Read the model definition and answer for the solid it produces. Units are mm, in the model's axes. A direction names the side the tool comes from. Round coordinates to 2 decimals unless told otherwise and drop trailing zeros. Order: outer loops, then holes, each group sorted by start corner. A loop starts at its lowest first (then second) coordinate and runs counter-clockwise, first axis right, second up. Notation, with made-up numbers: M 78,85.5 L 130,85.5 A18 ccw 130,114.5 Z; hole C 44.25,4 d4. An arc over 180 degrees is marked long. Use one line per item in the form item = value. Start each with the question number.
from build123d import *

# Parameters (mm, degrees)
BOSS_EXTRUDE1_DEPTH     = 5
CUT_EXTRUDE2_DEPTH      = 1
CUT_EXTRUDE2_DEPTH_BACK = 1
FILLET1_R               = 1
BOSS_EXTRUDE3_DEPTH     = 10
FILLET2_R               = 0.8


with BuildPart() as part:
    # Sketch1 → Boss-Extrude1 (new body)
    with BuildSketch(Plane(origin=(0, 0, 0), x_dir=(1, 0, 0), z_dir=(0, 1, 0))):
        with BuildLine():
            Line((-3.9, 3.9), (0, 3.9))
            ThreePointArc((0, 3.9), (2.757716447, 2.757716447), (3.9, 0))
            Line((3.9, 0), (3.9, -3.9))
            Line((3.9, -3.9), (0, -3.9))
            ThreePointArc((0, -3.9), (-2.757716447, -2.757716447), (-3.9, 0))
            Line((-3.9, 0), (-3.9, 3.9))
        make_face()
    extrude(amount=BOSS_EXTRUDE1_DEPTH)

    # Sketch3 → Cut-Extrude2 (cut, two sides: drawn at the far end of the back side and taken through both)
    with BuildSketch(Plane(origin=(0, 2.5, 0), x_dir=(1, 0, 0), z_dir=(0, 1, 0)).offset(-CUT_EXTRUDE2_DEPTH_BACK)):
        with BuildLine():
            Line((-3.9, 0), (-3.9, 3.9))
            Line((-3.9, 3.9), (0, 3.9))
            ThreePointArc((0, 3.9), (2.757716447, 2.757716447), (3.9, 0))
            Line((3.9, 0), (3.9, -3.9))
            Line((3.9, -3.9), (0, -3.9))
            ThreePointArc((0, -3.9), (-2.757716447, -2.757716447), (-3.9, 0))
        make_face()
        with BuildLine():
            Line((-2.9, 0), (-2.9, 2.9))
            Line((-2.9, 2.9), (0, 2.9))
            ThreePointArc((0, 2.9), (2.050609665, 2.050609665), (2.9, 0))
            Line((2.9, 0), (2.9, -2.9))
            Line((2.9, -2.9), (0, -2.9))
            ThreePointArc((0, -2.9), (-2.050609665, -2.050609665), (-2.9, 0))
        make_face(mode=Mode.SUBTRACT)
    extrude(amount=CUT_EXTRUDE2_DEPTH + CUT_EXTRUDE2_DEPTH_BACK, mode=Mode.SUBTRACT)

    # Fillet1
    fillet1_edges = [part.edges().sort_by_distance(p)[0] for p in [
        (2.9, 3.5, 1.45),
        (2.050609665, 3.5, -2.050609665),
        (1.45, 3.5, 2.9),
        (-2.050609665, 3.5, 2.050609665),
        (2.9, 1.5, 1.45),
        (2.050609665, 1.5, -2.050609665),
        (-2.9, 1.5, -1.45),
        (1.45, 1.5, 2.9),
        (-1.45, 3.5, -2.9),
        (-2.9, 3.5, -1.45),
        (-1.45, 1.5, -2.9),
        (-2.050609665, 1.5, 2.050609665),
    ]]
    fillet(fillet1_edges, radius=FILLET1_R - 0.0001)  # a hair under: the kernel refuses the full size

    # Sketch4 → Boss-Extrude3 (add)
    with BuildSketch(Plane(origin=(0, 5, 0), x_dir=(1, 0, 0), z_dir=(0, 1, 0))):
        with BuildLine():
            Line((0, 3.9), (-3.9, 3.9))
            Line((-3.9, 3.9), (-3.9, 0))
            ThreePointArc((-3.9, 0), (-2.757716447, -2.757716447), (0, -3.9))
            Line((0, -3.9), (3.9, -3.9))
            Line((3.9, -3.9), (3.9, 0))
            ThreePointArc((3.9, 0), (2.757716447, 2.757716447), (0, 3.9))
        make_face()
        with BuildLine():
            Line((-2.2627417, -0.565685425), (-0.565685425, -2.2627417))
            ThreePointArc((-0.565685425, -2.2627417), (0, -2.497056275), (0.565685425, -2.2627417))
            Line((0.565685425, -2.2627417), (2.2627417, -0.565685425))
            ThreePointArc((2.2627417, -0.565685425), (2.497056275, 0), (2.2627417, 0.565685425))
            Line((2.2627417, 0.565685425), (0.565685425, 2.2627417))
            ThreePointArc((0.565685425, 2.2627417), (0, 2.497056275), (-0.565685425, 2.2627417))
            Line((-0.565685425, 2.2627417), (-2.2627417, 0.565685425))
            ThreePointArc((-2.2627417, 0.565685425), (-2.497056275, 0), (-2.2627417, -0.565685425))
        make_face(mode=Mode.SUBTRACT)
    extrude(amount=BOSS_EXTRUDE3_DEPTH)

    # Fillet2
    fillet2_edges = [part.edges().sort_by_distance(p)[0] for p in [
        (0, 15, 2.497056275),
        (1.414213562, 15, 1.414213562),
        (2.497056275, 15, 0),
        (1.414213562, 15, -1.414213562),
        (0, 15, -2.497056275),
        (-1.414213562, 15, -1.414213562),
        (-2.497056275, 15, 0),
        (-1.414213562, 15, 1.414213562),
    ]]
    fillet(fillet2_edges, radius=FILLET2_R)


solid = part.part
Item 1: A tool of negligible diameter and unlimited length cuts with its end or side. For faces 4 (the cylindrical face through (3.201, 1.785, 1.544)), 5 (the cylindrical face through (-3.185, 3.199, -1.544)), 6 (the cylindrical face through (1.596, 14.772, 1.572)), from which of +Z, -Z, +X, -X, +Y, -Y can it reach the whole face along a straight path? Write none if from no direction.
Item 2: Find the intervals of material crossed by L1, parallel to Y at x = -3.5, z = -1.5; L2, parallel to X at y = 8.5, z = -0.25; L3, parallel to Y at x = -1.5, z = 2.75, in increasing order. Write a range as [from, to].
Item 3: Given P1, Ø2.5, axis at x = 0, z = -1, coming from the +Y side; P2, Ø1.5, axis at x = 1.5, z = -0.5, coming from the +Y side, each flat-ended and moving along its own axis, determine where each tip first touches the part or whether it passes through.
Item 4: Section A-A (y = 7.75) is taken. Write down the section's boundary in (x, z).
Item 5: Section B-B (y = 3) is taken. Write down the section's boundary in (x, z).
Item 6: For a pull along Z with two mould halves and no side action, classify faces 1 (the flat face through (-2, 9, -3.9)), 2 (the flat face through (-1.43, 9.54, 1.4)), 3 (the flat face through (-3.9, 1, -2)) as pulls with the +Z half, pulls with the -Z half, needs draft (parallel to the pull), parting line crosses it, or undercut.
The answers:
q1.face_4 = +Z, -Z, +X
q1.face_5 = +Z, -Z, -X
q1.face_6 = +Y
q2.L1 = [0, 1.58], [3.42, 15]
q2.L2 = [-3.9, -2.46], [2.46, 3.89]
q2.L3 = [0, 1.86], [3.14, 15]
q3.P1 = 5
q3.P2 = 14.69
q4.outline = M -3.9,-3.9 L 0,-3.9 A3.9 ccw 3.9,0 L 3.9,3.9 L 0,3.9 A3.9 ccw -3.9,0 Z; hole M -2.26,-0.57 L -0.57,-2.26 A0.8 ccw 0.57,-2.26 L 2.26,-0.57 A0.8 ccw 2.26,0.57 L 0.57,2.26 A0.8 ccw -0.57,2.26 L -2.26,0.57 A0.8 ccw Z
q5.outline = M -3.03,-3.03 L 0,-3.03 A3.03 ccw 3.03,0 L 3.03,3.03 L 0,3.03 A3.03 ccw -3.03,0 Z
q6.face_1 = pulls with the -Z half
q6.face_2 = undercut
q6.face_3 = needs draft
